Can you work these out from the drawing? Everything is in mm from the part's minimum corner. A direction names the side the tool comes from. Coordinates: 2 decimals unless noted, no trailing zeros. Order: outer loops, then holes, each group sorted by start corner. A loop starts at its lowest first (then second) coordinate and runs counter-clockwise, first axis right, second up. Notation, with made-up numbers: (-7.75, 72) -> (39.25, 72) arc R21 ccw to (39.25, 87) -> close; hole circle Ø3 at (81.5, -39.75). An arc over 180 degrees is marked (long way). Return JSON: item names as keys, results as strings. Group by question number.
1) Thinking about a two-plate mould opening in Y: for the marked faces 4, 5 and 6, which applies, +Y half, -Y half, draft (parallel to the pull), parting line (faces both ways), or undercut?
2) If we section it at C-C, the plane y = 6: Please give me the cut outline in (x, z), then the cut area to 3 significant figures.
3) If we section it at A-A, the plane x = 2.25: Please give me the cut outline in (y, z).
4) If I drill on probe 1 along Y at (x, z) = (12.25, 1.8); probe 2 along X at (y, z) = (9.25, 1.5), over which ranges is the centre line in solid material (lowest first)? Write a range as from..to.
5) For pin 1 (1.5 mm diameter, centred on x = 1, z = 2, fed in from -Y); pin 2 (1 mm diameter, centred on y = 4.5, z = 0.5, fed in from -X); pin 3 (1.5 mm diameter, centred on x = 11, z = 1, fed in from +Y), each with a flat end and sliding along its axis, tell me the tip position at first contact or that it passes through.
6) If we section it at B-B, the plane z = 2.45: Please give me the cut outline in (x, y), then the cut area to 3 significant figures.
7) For the marked faces 1, 2 and 3, which set-ups out of +Z, -Z, +X, -X, +Y, -Y let a thin tool reach every point of the face, with its end or its side?
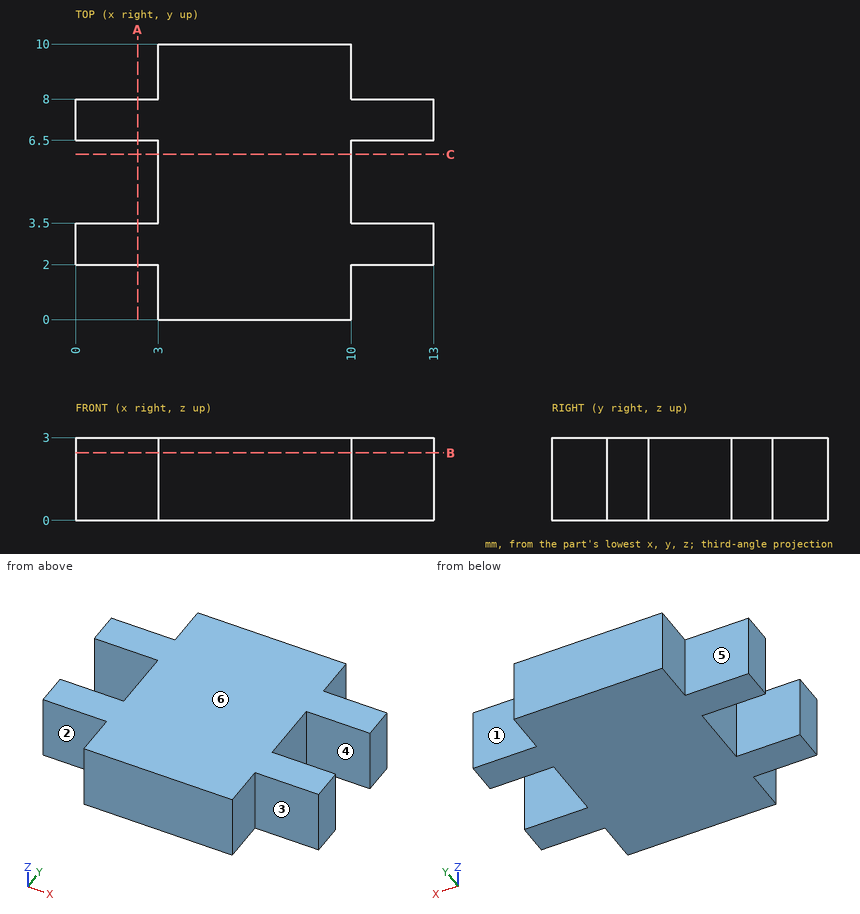
Result sheet:
{
 "1": {"face 4": "undercut", "face 5": "+Y half", "face 6": "draft"},
 "2": {"outline": "(3, 0) -> (10, 0) -> (10, 3) -> (3, 3) -> close", "area": "21.0 mm2"},
 "3": {"outline": "(2, 0) -> (3.5, 0) -> (3.5, 3) -> (2, 3) -> close; (6.5, 0) -> (8, 0) -> (8, 3) -> (6.5, 3) -> close"},
 "4": {"probe 1": "y = 2..3.5, 6.5..8", "probe 2": "x = 3..10"},
 "5": {"pin 1": "stops at y = 2", "pin 2": "stops at x = 3", "pin 3": "stops at y = 8"},
 "6": {"outline": "(0, 2) -> (3, 2) -> (3, 0) -> (10, 0) -> (10, 2) -> (13, 2) -> (13, 3.5) -> (10, 3.5) -> (10, 6.5) -> (13, 6.5) -> (13, 8) -> (10, 8) -> (10, 10) -> (3, 10) -> (3, 8) -> (0, 8) -> (0, 6.5) -> (3, 6.5) -> (3, 3.5) -> (0, 3.5) -> close", "area": "88.0 mm2"},
 "7": {"face 1": "+Z, -Z, +X, +Y", "face 2": "+Z, -Z, -X, -Y", "face 3": "+Z, -Z, +X, -Y"}
}
